The drawing under review shows one solid part. Ordinate dimensions are in mm from its lowest x, y, z. A direction names the side the tool comes from. Give positions to 0.01 mm unless a question says otherwise; leave off trailing zeros. Order: outer loops, then holes, each group sorted by start corner. A loop starts at its lowest first (then second) coordinate and runs counter-clockwise, first axis right, second up. Notation, with made-up numbers: (-31.75, -2.5) - (6.25, -2.5) arc R20 cw to (6.25, 23.5) - close; hole circle Ø7 at (-28, 78.5). An arc over 180 degrees is marked (long way). Use CSV: the item, a comma, the result in double quotes. Start each with the question number.
1. Take a section at B-B, the plane y = 36.5. State the section outline as (x, z) points (1 decimal).
2. To check wall thickness, follow line 1 (X direction, y = 40.5, z = 25.5) (1 decimal). State the ranges of the line that lie inside material, in increasing order. Write a range as [from, to].
3. For pin 1 (3 mm diameter, centred on y = 41.275, z = 9.525, fed in from -X); pin 2 (5 mm diameter, centred on y = 17, z = 56.5, fed in from +X) (3 decimals); pin 3 (2 mm diameter, centred on y = 12, z = 91.5, fed in from -X); pin 4 (2 mm diameter, centred on x = 19, z = 44, fed in from +Y) (3 decimals), all flat-tipped, find the tip position at first contact; note any pin that passes through.
4. Take a section at A-A, the plane z = 44. State the section outline as (x, y) points (1 decimal).
5. Take a section at C-C, the plane x = 12. State the section outline as (y, z) points (1 decimal), then the cut area to 3 significant figures.
6. Machinability: for the marked faces 1 and 2, which of the approach directions +Z, -Z, +X, -X, +Y, -Y give a long, thin tool a straight path to every point of the face, cutting with its end or side? Answer none if there is none.
7. Take a section at D-D, the plane z = 105.5. State the section outline as (x, y) points (1 decimal).
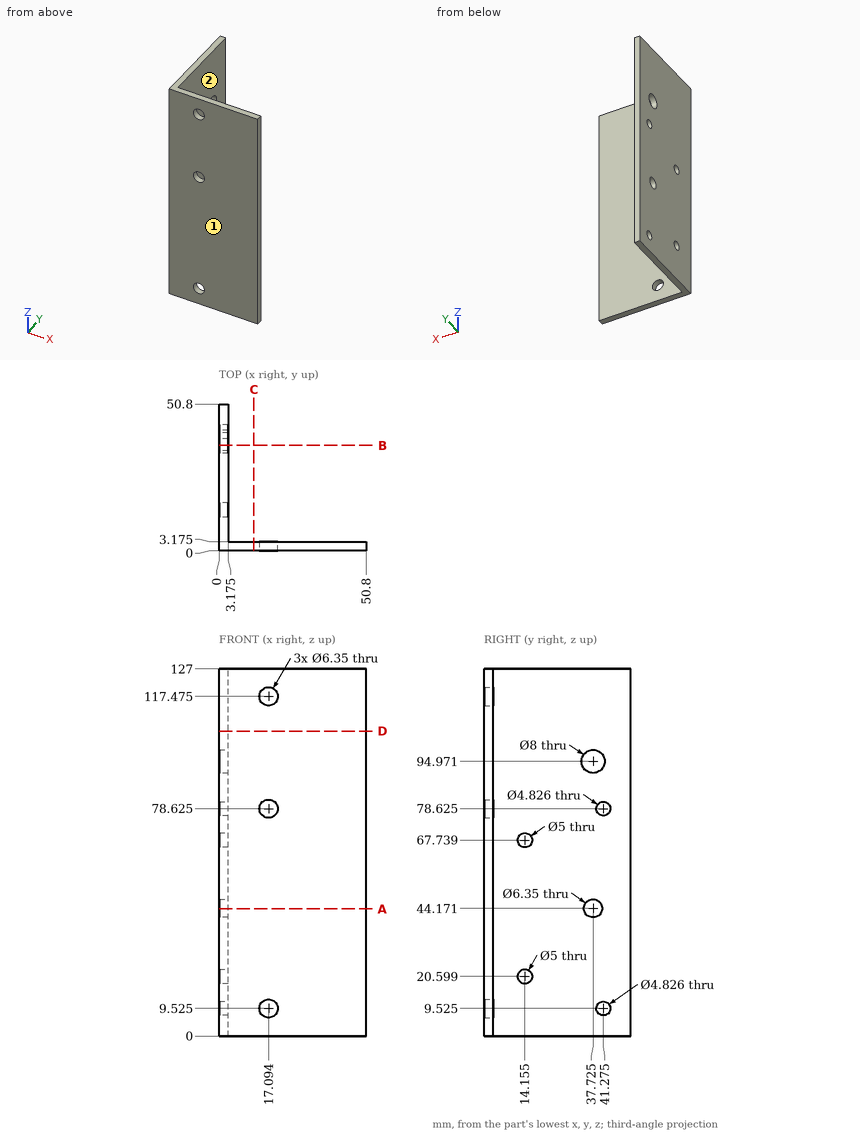
Determined:
1,outline,"(0, 0) - (3.2, 0) - (3.2, 41.2) - (0, 41.2) - close; (0, 47.1) - (3.2, 47.1) - (3.2, 91.2) - (0, 91.2) - close; (0, 98.8) - (3.2, 98.8) - (3.2, 127) - (0, 127) - close"
2,line 1,"x = [0, 3.2]"
3,pin 1,"passes through"
3,pin 2,"stops at x = 3.175"
3,pin 3,"stops at x = 0"
3,pin 4,"stops at y = 3.175"
4,outline,"(0, 0) - (50.8, 0) - (50.8, 3.2) - (3.2, 3.2) - (3.2, 34.6) - (0, 34.6) - close; (0, 40.9) - (3.2, 40.9) - (3.2, 50.8) - (0, 50.8) - close"
5,outline,"(0, 0) - (3.2, 0) - (3.2, 127) - (0, 127) - close"
5,area,"403 mm²"
6,face 1,"+Z, -Z, +X, -X, -Y"
6,face 2,"+Z, -Z, +X, +Y"
7,outline,"(0, 0) - (50.8, 0) - (50.8, 3.2) - (3.2, 3.2) - (3.2, 50.8) - (0, 50.8) - close"
